Answer from the drawing. Dimensions are ordinates in mm from the lowest x, y and z of the part. A direction names the side the tool comes from. Coordinates: 2 decimals unless noted, no trailing zeros. Write each loop counter-clockwise with the first axis right and the second up, starting at its lowest first coordinate (ties: lowest second). Pieces come first, ordered by that corner, then holes.
(1) Which of the six approach directions +Z, -Z, +X, -X, +Y, -Y give full straight-line access (tool end or side, diameter ignored) to the marked faces 1, 2 and 3?
(2) The part is cut by section A-A, the plane x = 30. Determine the outline of the cut face in (y, z), and give its area (3 significant figures).
(3) Given pin 1 (3 mm diameter, centred on x = 5, y = 22.5, fed in from -Z); pin 2 (4.5 mm diameter, centred on x = 5, y = 7.5, fed in from +Z); pin 3 (1 mm diameter, centred on x = 10, y = 9, fed in from -Z); pin 4 (9 mm diameter, centred on x = 28.5, y = 22, fed in from +Z), each flat-ended and moving along its own axis, determine where each tip first touches the part or whether it passes through.
(4) Straight lines are drawn through the part: line 1 along Y through (x, z) = (5, 4.55); line 2 along Y through (x, z) = (5, 6); line 3 along Z through (x, y) = (12, 14). For each, find the intervals that lie inside material, in ascending order.
(5) The part is cut by section C-C, the plane x = 5. Determine the outline of the cut face in (y, z).
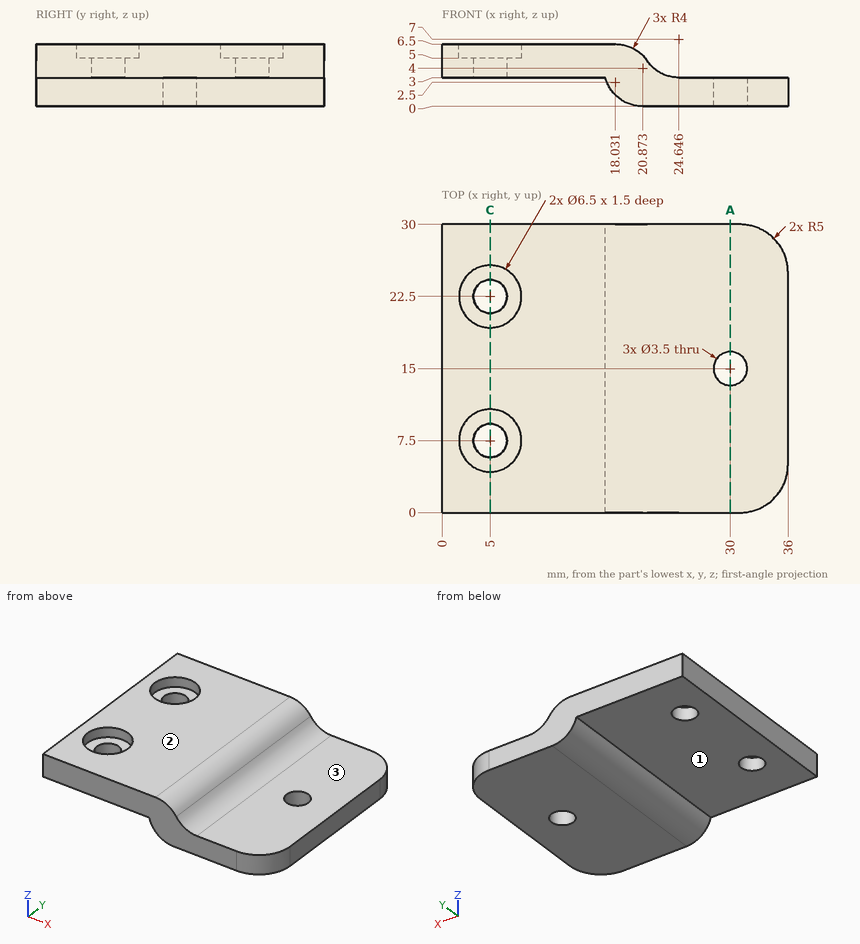
Computed:
1. face 1: -Z, -X, +Y, -Y
1. face 2: +Z, +X, -X, +Y, -Y
1. face 3: +Z, +X, +Y, -Y
2. outline: (0, 0) - (13.25, 0) - (13.25, 3) - (0, 3) - close; (16.75, 0) - (30, 0) - (30, 3) - (16.75, 3) - close
2. area: 79.5 mm2
3. pin 1: passes through
3. pin 2: stops at z = 5
3. pin 3: stops at z = 3
3. pin 4: stops at z = 3.05
4. line 1: y = 0 to 5.75, 9.25 to 20.75, 24.25 to 30
4. line 2: y = 0 to 4.25, 10.75 to 19.25, 25.75 to 30
4. line 3: z = 3 to 6.5
5. outline: (0, 3) - (5.75, 3) - (5.75, 5) - (4.25, 5) - (4.25, 6.5) - (0, 6.5) - close; (9.25, 3) - (20.75, 3) - (20.75, 5) - (19.25, 5) - (19.25, 6.5) - (10.75, 6.5) - (10.75, 5) - (9.25, 5) - close; (24.25, 3) - (30, 3) - (30, 6.5) - (25.75, 6.5) - (25.75, 5) - (24.25, 5) - close
